Part model, mm, in its own coordinate system. Face numbers are marked on the shaded views. Coordinates: 2 decimals unless noted, no trailing zeros. Order: outer loops, then holes, each group sorted by start corner. A loop starts at its lowest first (then second) coordinate and runs counter-clockwise, first axis right, second up. Notation, with made-up numbers: M -14,-14 L 26,-14 A24 cw 26,2 Z; hole C 68,64 d7. An arc over 180 degrees is marked long. Answer in a Markdown table with one row per item. Add a question column.
from build123d import *

# Parameters (mm, degrees)
SKETCH7_W           = 20
SKETCH7_H           = 40
SKETCH7_R           = 3.75
BOSS_EXTRUDE4_DEPTH = 20
SKETCH8_R           = 2.5
BOSS_EXTRUDE5_DEPTH = 20


with BuildPart() as part:
    # Sketch7 → Boss-Extrude4 (new body)
    with BuildSketch(Plane.XY):
        with Locations((10, 20)):
            Rectangle(SKETCH7_W, SKETCH7_H)
        with Locations((15, 7.90672248)):
            Circle(SKETCH7_R, mode=Mode.SUBTRACT)
        with Locations((5, 7.90672248)):
            Circle(SKETCH7_R, mode=Mode.SUBTRACT)
        with Locations((9.590015998, 32.1)):
            Circle(SKETCH7_R, mode=Mode.SUBTRACT)
    extrude(amount=BOSS_EXTRUDE4_DEPTH)

    # Sketch8 → Boss-Extrude5 (add)
    with BuildSketch(Plane(origin=(20, 0, 0), x_dir=(0, 0, -1), z_dir=(1, 0, 0))):
        with Locations(Location((-10, 29.176257045, 0), (0, 0, 180))):
            Circle(SKETCH8_R)
    extrude(amount=BOSS_EXTRUDE5_DEPTH)


solid = part.part
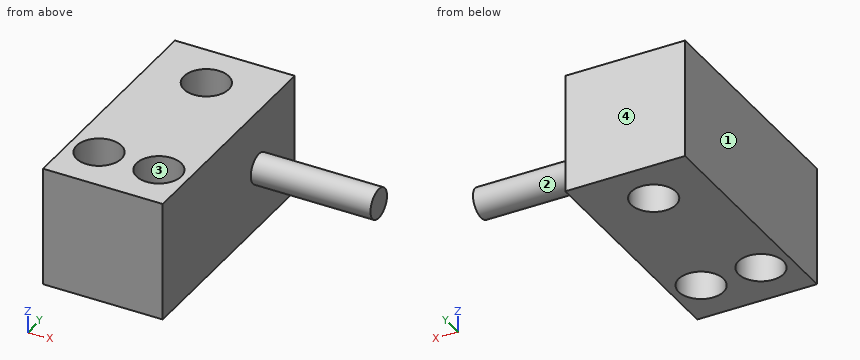
(1) Slice it at A-A (x = 5). List the corners of the cut face in (y, z).
(2) Slice it at B-B (z = 5). List the corners of the cut face in (x, y).
(3) Drop flat-ended pins along their axis: P1, Ø6, axis at x = 9.59, y = 32.1, coming from the +Z side; P2, Ø4, axis at y = 10.5, z = 16.5, coming from the +X side; P3, Ø2, axis at x = 22.5, y = 28, coming from the -Z side. Give the stop position or say it passes through.
(4) Pull direction Y, two halves, no side cores. Call the marked faces 1, 2, 3 and 4: pulls with the +Y half, pulls with the -Y half, needs draft (parallel to the pull), parting line crosses it, or undercut.
(5) Wall check: line 1 (Y direction, x = 15, z = 12.25); line 2 (X direction, y = 18.5, z = 5.75); line 3 (Y direction, x = 7.5, z = 11). Give the ranges that are in metal, low to high.
(6) Slice it at C-C (y = 24.5). List the corners of the cut face in (x, z), and give its area (3 significant figures).
(7) Slice it at D-D (x = 12). List the corners of the cut face in (y, z), and give its area (3 significant figures).
Computed:
| question | item | result |
|---|---|---|
| 1 | outline | M 0,0 L 4.16,0 L 4.16,20 L 0,20 Z; M 11.66,0 L 40,0 L 40,20 L 11.66,20 Z |
| 2 | outline | M 0,0 L 20,0 L 20,40 L 0,40 Z; hole C 5,7.91 d7.5; hole C 9.59,32.1 d7.5; hole C 15,7.91 d7.5 |
| 3 | P1 | passes through |
| 3 | P2 | stops at x = 20 |
| 3 | P3 | stops at z = 7.51 |
| 4 | face 1 | needs draft |
| 4 | face 2 | parting line crosses it |
| 4 | face 3 | undercut |
| 4 | face 4 | pulls with the +Y half |
| 5 | line 1 | y = 0 to 4.16, 11.66 to 40 |
| 5 | line 2 | x = 0 to 20 |
| 5 | line 3 | y = 0 to 5.11, 10.7 to 28.99, 35.21 to 40 |
| 6 | outline | M 0,0 L 20,0 L 20,20 L 0,20 Z |
| 6 | area | 400 mm^2 |
| 7 | outline | M 0,0 L 5.66,0 L 5.66,20 L 0,20 Z; M 10.16,0 L 29.23,0 L 29.23,20 L 10.16,20 Z; M 34.97,0 L 40,0 L 40,20 L 34.97,20 Z |
| 7 | area | 595 mm^2 |
